The listing builds one solid part. Answer for the finished solid, in the listing's coordinates (mm). A direction names the side the tool comes from. Give positions to 0.01 mm unless a question says otherwise; leave off trailing zeros. Loops run counter-clockwise (first coordinate to the right, second up) from the corner with the lowest first, then second, coordinate; pieces in that order, holes last. Notation, with made-up numbers: (61.5, -10) - (108.5, -10) arc R4 cw to (108.5, -3) - close; hole circle Ø10 at (40.25, 81). An arc over 180 degrees is marked (long way). Answer as CSV lines item,"result". Start each with the question number.
1) A cutting plane is placed at A-A (y = -10.25). Determine the outline of the cut face in (x, z).
2) Find the intervals of material crossed by line 1 along Y through (x, z) = (-37.5, 2); line 2 along Y through (x, z) = (-39.5, 0.5); line 3 along X through (y, z) = (-6.5, 3.25), in increasing order.
3) A cutting plane is placed at C-C (y = 11.5). Determine the outline of the cut face in (x, z).
4) For a pull along Y with two mould halves and no side action, classify faces 4 (the face through (60.3, -9.87, 3.04)), 5 (the face through (11.6, 7.83, 1.48)), 6 (the face through (-33, -5, 0)) as pulls with the +Y half, pulls with the -Y half, needs draft (parallel to the pull), parting line crosses it, or undercut.
5) Flat-ended cylindrical pins translate along their axes: pin 1 (0.9 mm diameter, centred on x = 12.5, y = 21, fed in from -Z); pin 2 (19 mm diameter, centred on x = 30, y = -22, fed in from -Z); pin 3 (3.5 mm diameter, centred on x = -55, y = -2, fed in from +Z); pin 4 (1 mm diameter, centred on y = -20.5, z = 5, fed in from +X). Find the tip coordinate at first contact, or state that the pin passes through.
6) A cutting plane is placed at B-B (x = 38.5). Determine the outline of the cut face in (y, z), and give its area (3 significant figures).
7) For faces 1 (the face through (12, 20, 1.5)), 2 (the face through (-55, -9, 3)), 3 (the face through (-41, -40, 1)), determine the directions among +Z, -Z, +X, -X, +Y, -Y from which every point of the face is accessible in a straight line to the end or side of a thin tool.
```python
from build123d import *

# Parameters (mm, degrees)
SKETCH_1_W           = 130
SKETCH_1_H           = 60
EXTRUDE_1_DEPTH      = 6
EXTRUDE_2_DEPTH      = 3
EXTRUDE_2_DEPTH_BACK = 133
SKETCH_2_W           = 3
SKETCH_2_H           = 60
SKETCH_3_R           = 1.25
SKETCH_3_W           = 5
SKETCH_3_H           = 16
SKETCH_3_W_2         = 40
SKETCH_3_H_2         = 10
SKETCH_3_W_3         = 34
CUT_EXTRUDE_1_DEPTH  = 6
CUT_EXTRUDE_2_DEPTH  = 1.5
SKETCH_5_W           = 70
SKETCH_5_H           = 41.476582403
SKETCH_5_W_2         = 24
SKETCH_5_H_2         = 16
CUT_EXTRUDE_3_DEPTH  = 3
CHAMFER_1_SIZE       = 15
CHAMFER_1_SIZE_2     = 3
CUT_EXTRUDE_4_DEPTH  = 3
SKETCH_7_W           = 130
SKETCH_7_H           = 1.5
EXTRUDE_3_DEPTH      = 3


with BuildPart() as part:
    # 草圖1 → 填料-伸長1 (new body)
    with BuildSketch(Plane.XY):
        with Locations((11.111111111, -11.25)):
            Rectangle(SKETCH_1_W, SKETCH_1_H)
    extrude(amount=EXTRUDE_1_DEPTH)

    # 草圖2 → 填料-伸長2 (add, two sides: drawn at the far end of the back side and taken through both)
    with BuildSketch(Plane.ZY.offset(53.888888889).offset(-EXTRUDE_2_DEPTH_BACK)):
        with Locations((1.5, -11.25)):
            Rectangle(SKETCH_2_W, SKETCH_2_H)
    extrude(amount=EXTRUDE_2_DEPTH + EXTRUDE_2_DEPTH_BACK)

    # 草圖3 → 除料-伸長1 (cut)
    with BuildSketch(Plane.XY.offset(6)):
        with Locations((59.111111111, -10.25)):
            Circle(SKETCH_3_R)
        with Locations((-50.388888889, -10.25)):
            Circle(SKETCH_3_R)
        with Locations((72.611111111, -26.75)):
            Rectangle(SKETCH_3_W, SKETCH_3_H)
        with Locations((-26.888888889, -10.75)):
            Rectangle(SKETCH_3_W_2, SKETCH_3_H_2)
        with Locations((27.111111111, -10.75)):
            Rectangle(SKETCH_3_W_3, SKETCH_3_H_2)
    extrude(amount=-CUT_EXTRUDE_1_DEPTH, mode=Mode.SUBTRACT)

    # 草圖4 → 除料-伸長2 (cut)
    with BuildSketch(Plane.XY.offset(6)):
        with BuildLine():
            Line((5.161633763, -27.924686511), (3.254050898, -27.924686511))
            add(Edge.make_bspline(
                [(3.254050898, -27.924686511), (3.192249579, -27.924078509), (3.072379909, -27.922899232), (2.898729115, -27.915701709), (2.736761533, -27.904944526), (2.586564336, -27.888174414), (2.448251756, -27.865582926), (2.322097886, -27.838909636), (2.207853822, -27.808266207), (2.105836262, -27.771295953), (2.01510686, -27.730787239), (1.936069122, -27.68581143), (1.86982721, -27.634270004), (1.815766676, -27.57730265), (1.772168095, -27.516260775), (1.742170993, -27.449388735), (1.72280295, -27.378127045), (1.720982885, -27.328575874), (1.72005993, -27.303448471)],
                knots=[0, 0, 0, 0, 1.637449122, 3.175991815, 4.604285445, 5.937552174, 7.178588142, 8.315988927, 9.352959284, 10.309701018, 11.187868748, 11.983148269, 12.713194599, 13.402748524, 14.058038132, 14.690029686, 15.335713943, 16, 16, 16, 16], degree=3))
            add(Edge.make_bspline(
                [(1.72005993, -27.303448471), (1.723635689, -27.258199951), (1.731180344, -27.162728075), (1.787663263, -27.019644469), (1.87219849, -26.869087652), (1.94824443, -26.77316), (1.988932886, -26.721833814)],
                knots=[0, 0, 0, 0, 0.830703556, 1.752738595, 2.797600559, 4, 4, 4, 4], degree=3))
            add(Edge.make_bspline(
                [(1.988932886, -26.721833814), (2.063514276, -26.639331654), (2.213358857, -26.473573125), (2.362577426, -26.307250824), (2.437526185, -26.223711286)],
                knots=[0, 0, 0, 0, 0.995449954, 2, 2, 2, 2], degree=3))
            add(Edge.make_bspline(
                [(2.437526185, -26.223711286), (2.47103383, -26.177024109), (2.540031377, -26.080887817), (2.64617827, -25.932308493), (2.757969515, -25.7748922), (2.87632458, -25.60941735), (3.003450981, -25.437027126), (3.133736422, -25.254119028), (3.273689868, -25.064815864), (3.417008587, -24.865483968), (3.567026655, -24.658540826), (3.724948502, -24.444530992), (3.888719581, -24.221478696), (4.058065694, -23.989527198), (4.234458829, -23.749756028), (4.416012984, -23.500904526), (4.606300307, -23.245131026), (4.734336909, -23.071345188), (4.799362833, -22.983084609)],
                knots=[0, 0, 0, 0, 0.68787784, 1.416449417, 2.185717103, 2.998962895, 3.851631247, 4.749555124, 5.686911444, 6.669516273, 7.688234189, 8.746402434, 9.853137794, 11.000549032, 12.184081851, 13.416182313, 14.687757029, 16, 16, 16, 16], degree=3))
            add(Edge.make_bspline(
                [(4.799362833, -22.983084609), (4.830971294, -22.943553506), (4.892623413, -22.866448317), (4.999342936, -22.767074964), (5.111072502, -22.681126787), (5.230934533, -22.611368569), (5.358194037, -22.556625494), (5.493063713, -22.519613637), (5.634235505, -22.493643771), (5.730861536, -22.49164161), (5.780041561, -22.490622564)],
                knots=[0, 0, 0, 0, 1.06425237, 2.0758181, 3.06095989, 4.026690108, 4.987711416, 5.968488933, 6.966016048, 8, 8, 8, 8], degree=3))
            add(Edge.make_bspline(
                [(5.780041561, -22.490622564), (5.826442291, -22.491944732), (5.916313772, -22.494505581), (6.045628911, -22.523235489), (6.166636791, -22.565562498), (6.23827235, -22.610014837), (6.273918727, -22.632134646)],
                knots=[0, 0, 0, 0, 1.066082933, 2.064847948, 3.037054213, 4, 4, 4, 4], degree=3))
            add(Edge.make_bspline(
                [(6.273918727, -22.632134646), (6.311441096, -22.661555246), (6.384541176, -22.718871676), (6.465186438, -22.833465288), (6.511587665, -22.966478607), (6.517237732, -23.060547629), (6.52014975, -23.109030362)],
                knots=[0, 0, 0, 0, 1.018925786, 1.985044098, 2.961501162, 4, 4, 4, 4], degree=3))
            Line((6.52014975, -23.109030362), (6.52014975, -26.656738256))
            add(Edge.make_bspline(
                [(6.52014975, -26.656738256), (6.571120358, -26.658160603), (6.668428141, -26.660876), (6.807468472, -26.672045587), (6.933741535, -26.681782224), (7.04627481, -26.698396225), (7.146439706, -26.713806583), (7.232355911, -26.736203852), (7.306925886, -26.756584321), (7.349633605, -26.777387591), (7.369222241, -26.786929372)],
                knots=[0, 0, 0, 0, 1.415561033, 2.70244186, 3.872869685, 4.930574004, 5.860813375, 6.683597148, 7.396208987, 8, 8, 8, 8], degree=3))
            add(Edge.make_bspline(
                [(7.369222241, -26.786929372), (7.387933285, -26.798727315), (7.425308471, -26.82229363), (7.475291838, -26.865642335), (7.515332971, -26.918922636), (7.550217281, -26.978243638), (7.574189335, -27.047295447), (7.595611952, -27.122551217), (7.603742149, -27.206589411), (7.605862425, -27.264770318), (7.606962539, -27.294957746)],
                knots=[0, 0, 0, 0, 0.898852474, 1.795451925, 2.670043032, 3.597686986, 4.580760669, 5.631985542, 6.771344949, 8, 8, 8, 8], degree=3))
            add(Edge.make_bspline(
                [(7.606962539, -27.294957746), (7.6065918, -27.327130489), (7.605877096, -27.389152557), (7.587829145, -27.478153146), (7.560306222, -27.5599435), (7.518416649, -27.632950045), (7.464991439, -27.697675729), (7.400296134, -27.754477063), (7.324655873, -27.805253805), (7.267343492, -27.829851085), (7.237616005, -27.842609503)],
                knots=[0, 0, 0, 0, 1.087494211, 2.096452886, 3.061576041, 3.998924861, 4.929714891, 5.891658933, 6.906419893, 8, 8, 8, 8], degree=3))
            add(Edge.make_bspline(
                [(7.237616005, -27.842609503), (7.190336116, -27.858712295), (7.089569557, -27.893031811), (6.919845265, -27.915756431), (6.72799274, -27.93166309), (6.591892116, -27.927094657), (6.52014975, -27.924686511)],
                knots=[0, 0, 0, 0, 0.822901404, 1.753831169, 2.815982903, 4, 4, 4, 4], degree=3))
            add(Edge.make_bspline(
                [(6.52014975, -27.924686511), (6.52249173, -28.040722435), (6.52728009, -28.27796686), (6.525874109, -28.640744347), (6.523902436, -29.018132536), (6.518606285, -29.274244271), (6.515904387, -29.404902888)],
                knots=[0, 0, 0, 0, 0.940774337, 1.923485917, 2.940640271, 4, 4, 4, 4], degree=3))
            add(Edge.make_bspline(
                [(6.515904387, -29.404902888), (6.513253145, -29.446642645), (6.508069894, -29.528245001), (6.47349895, -29.644606371), (6.416416736, -29.749022953), (6.340813008, -29.84091244), (6.245918419, -29.915035809), (6.135823145, -29.970814241), (6.008973806, -30.001054572), (5.919815256, -30.005455315), (5.873439535, -30.007744357)],
                knots=[0, 0, 0, 0, 1.014791907, 1.983945634, 2.923310284, 3.892735559, 4.856647083, 5.831419924, 6.872015472, 8, 8, 8, 8], degree=3))
            add(Edge.make_bspline(
                [(5.873439535, -30.007744357), (5.815037496, -30.005688173), (5.704234702, -30.001787096), (5.550592692, -29.954784505), (5.418967159, -29.880845956), (5.316601579, -29.770806418), (5.237109991, -29.634349624), (5.185909967, -29.467148659), (5.160681119, -29.271746214), (5.161303076, -29.132326216), (5.161633763, -29.058198287)],
                knots=[0, 0, 0, 0, 1.02325021, 1.941353164, 2.796047092, 3.646386069, 4.549425683, 5.551115642, 6.69795776, 8, 8, 8, 8], degree=3))
            Line((5.161633763, -29.058198287), (5.161633763, -27.924686511))
        make_face()
        with BuildLine():
            add(Edge.make_bspline(
                [(5.161633763, -24.57368041), (5.119646014, -24.636412887), (5.031158393, -24.768619255), (4.891120499, -24.978124945), (4.731778952, -25.205824972), (4.560305824, -25.457296058), (4.369434267, -25.726531763), (4.166450797, -26.019598708), (3.9439664, -26.33065406), (3.791254445, -26.545837446), (3.712550044, -26.656738256)],
                knots=[0, 0, 0, 0, 0.713938416, 1.50459871, 2.383225934, 3.342268853, 4.38315458, 5.504445422, 6.71384576, 8, 8, 8, 8], degree=3))
            Line((3.712550044, -26.656738256), (5.161633763, -26.656738256))
            Line((5.161633763, -26.656738256), (5.161633763, -24.57368041))
        make_face(mode=Mode.SUBTRACT)
    extrude(amount=-CUT_EXTRUDE_2_DEPTH, mode=Mode.SUBTRACT)

    # 草圖5 → 除料-伸長3 (cut)
    with BuildSketch(Plane(origin=(0, 0, 0), x_dir=(-1, 0, 0), z_dir=(0, 0, -1))):
        with Locations((-11.111111111, -20.511708798)):
            Rectangle(SKETCH_5_W, SKETCH_5_H)
        with Locations((-58.111111111, -26.75)):
            Rectangle(SKETCH_5_W_2, SKETCH_5_H_2)
    extrude(amount=-CUT_EXTRUDE_3_DEPTH, mode=Mode.SUBTRACT)

    # 導角1
    # the kernel refuses this chamfer: 15, 3 mm, written as the material it takes off along each edge
    with BuildSketch(Plane(origin=(46.111111111, 0.226582403, 0), x_dir=(0, 0.9999715107910818, -0.00754835122404063), z_dir=(-1, 0, 0))) as chamfer_1_piece_1_section:
        Polygon((CHAMFER_1_SIZE * 0.999971510791, -CHAMFER_1_SIZE * 0.00754835122404), (-CHAMFER_1_SIZE_2 * 0.00754835122404, -CHAMFER_1_SIZE_2 * 0.999971510791), (0, 0), align=None)
    chamfer_1_piece_1 = extrude(amount=70, mode=Mode.PRIVATE)
    chamfer_1_piece_1 = split(chamfer_1_piece_1, bisect_by=Plane(origin=(11.111111111, 5.568156657, 3), z_dir=(0, 0, -1)), keep=Keep.TOP, mode=Mode.PRIVATE)
    add(chamfer_1_piece_1, mode=Mode.SUBTRACT)

    # 草圖6 → 除料-伸長4 (cut)
    with BuildSketch(Plane.XZ.offset(41.25)):
        Polygon((-53.888888889, 3), (-23.888888889, 3), (46.111111111, 3), (76.111111111, 3), (76.111111111, 5), (-53.888888889, 5), align=None)
        Polygon((-56.888888889, 3), (-56.888888889, 1), (-23.888888889, 1), (-23.888888889, 3), (-53.888888889, 3), align=None)
        Polygon((46.111111111, 3), (46.111111111, 1), (79.111111111, 1), (79.111111111, 3), (76.111111111, 3), align=None)
    extrude(amount=-CUT_EXTRUDE_4_DEPTH, mode=Mode.SUBTRACT)

    # 草圖7 → 填料-伸長3 (add)
    with BuildSketch(Plane(origin=(0, 18.75, 0), x_dir=(1, 0, 0), z_dir=(0, 1, 0))):
        Polygon((79.111111111, -1.5), (-56.888888889, -1.5), (-56.888888889, -3), (-53.888888889, -3), (76.111111111, -3), (79.111111111, -3), align=None)
        with Locations((11.111111111, -3.75)):
            Rectangle(SKETCH_7_W, SKETCH_7_H)
    extrude(amount=EXTRUDE_3_DEPTH)


solid = part.part
```
Ans:
1,outline,"(-56.89, 0) - (-51.64, 0) - (-51.64, 6) - (-53.89, 6) - (-53.89, 3) - (-56.89, 3) - close; (-49.14, 0) - (-46.89, 0) - (-46.89, 6) - (-49.14, 6) - close; (-6.89, 3) - (10.11, 3) - (10.11, 6) - (-6.89, 6) - close; (44.11, 3) - (46.11, 3) - (46.11, 0) - (57.86, 0) - (57.86, 6) - (44.11, 6) - close; (60.36, 0) - (79.11, 0) - (79.11, 3) - (76.11, 3) - (76.11, 6) - (60.36, 6) - close"
2,line 1,"-38.25 to -15.75, -5.75 to 21.75"
2,line 2,"-41.25 to -15.75, -5.75 to 18.75"
2,line 3,"-53.89 to -46.89, -6.89 to 10.11, 44.11 to 76.11"
3,outline,"(-56.89, 0) - (-23.89, 0) - (-23.89, 0.75) - (46.11, 0.75) - (46.11, 0) - (79.11, 0) - (79.11, 3) - (76.11, 3) - (76.11, 6) - (-53.89, 6) - (-53.89, 3) - (-56.89, 3) - close"
4,face 4,"undercut"
4,face 5,"pulls with the -Y half"
4,face 6,"needs draft"
5,pin 1,"z = 1.5"
5,pin 2,"z = 3"
5,pin 3,"z = 6"
5,pin 4,"x = 76.11"
6,outline,"(-41.25, 5) - (-38.25, 5) - (-38.25, 3) - (-15.75, 3) - (-15.75, 6) - (-41.25, 6) - close; (-5.75, 3) - (0.23, 3) - (15.23, 0) - (18.75, 0) - (18.75, 1.5) - (21.75, 1.5) - (21.75, 4.5) - (18.75, 4.5) - (18.75, 6) - (-5.75, 6) - close"
6,area,"186 mm2"
7,face 1,"-Z, +X, -X, +Y"
7,face 2,"+Z, -X, +Y, -Y"
7,face 3,"+X, -X, -Y"
